Source: CAD feature listing. Evaluate the final solid. Frame: model axes, mm. Face numbers are marked on the shaded views. Give positions to 0.01 mm unless a question says otherwise; leave off trailing zeros. Loops run counter-clockwise (first coordinate to the right, second up) from the corner with the lowest first, then second, coordinate; pieces in that order, holes last.
from build123d import *

# Parameters (mm, degrees)
SKETCH1_R           = 1.5
SKETCH1_R_2         = 1.75
SKETCH1_R_3         = 1.45
BOSS_EXTRUDE1_DEPTH = 15


with BuildPart() as part:
    # Sketch1 → Boss-Extrude1 (new body)
    with BuildSketch(Plane(origin=(0, 0, 0), x_dir=(1, 0, 0), z_dir=(0, 1, 0))):
        with BuildLine():
            ThreePointArc((-2.52975, 1.612564708), (-7.95, 0), (-2.52975, -1.612564708))
            ThreePointArc((-2.52975, -1.612564708), (-0.159877177, -2.995736852), (2.34375, -1.872654783))
            ThreePointArc((2.34375, -1.872654783), (8.25, 0), (2.34375, 1.872654783))
            ThreePointArc((2.34375, 1.872654783), (-0.159877177, 2.995736852), (-2.52975, 1.612564708))
        make_face()
        with Locations(Location((0, 0, 0), (0, 0, 270))):
            Circle(SKETCH1_R, mode=Mode.SUBTRACT)
        with Locations(Location((5, 0, 0), (0, 0, 270))):
            Circle(SKETCH1_R_2, mode=Mode.SUBTRACT)
        with Locations(Location((-5, 0, 0), (0, 0, 270))):
            Circle(SKETCH1_R_3, mode=Mode.SUBTRACT)
    extrude(amount=BOSS_EXTRUDE1_DEPTH)


solid = part.part
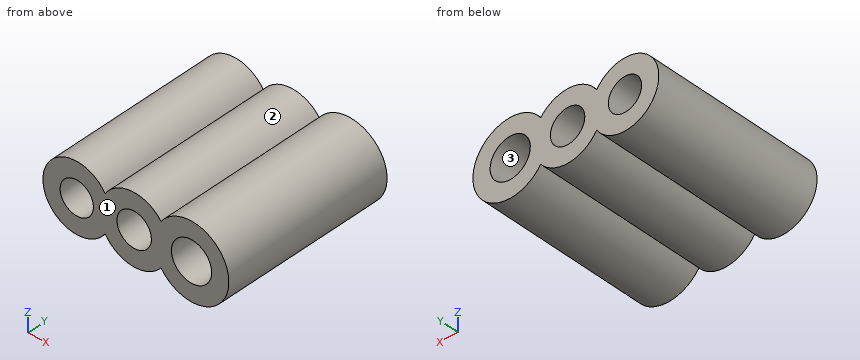
1) Cut plane C-C (y = 3). Return loops of the section in (x, z).
Checks:
outline: (-2.53, -1.61) arc R3 ccw to (2.34, -1.87) arc R3.25 ccw (long way) to (2.34, 1.87) arc R3 ccw to (-2.53, 1.61) arc R2.95 ccw (long way) to start; hole circle Ø2.9 at (-5, 0); hole circle Ø3 at (0, 0); hole circle Ø3.5 at (5, 0)
2) Ray query, probe 1 along X at (y, z) = (3.75, 0); probe 2 along X at (y, z) = (6.75, 1.25); probe 3 along X at (y, z) = (14, 2.25). Return the intervals inside material, ascending.
Checks:
probe 1: x = -7.95 to -6.45, -3.55 to -1.5, 1.5 to 3.25, 6.75 to 8.25
probe 2: x = -7.67 to -5.73, -4.27 to -0.83, 0.83 to 3.78, 6.22 to 8
probe 3: x = -6.91 to -3.09, -1.98 to 1.98, 2.65 to 7.35
3) Pull-direction query (X, two-part tool) for the marked faces 1, 2 and 3; classes: released by +X, released by -X, zero draft, split by the parting line, or undercut.
Checks:
face 1: zero draft
face 2: undercut
face 3: undercut
4) Cut plane B-B (z = 0). Return loops of the section in (x, y), and give its area (3 significant figures).
Checks:
outline: (-7.95, 0) - (-6.45, 0) - (-6.45, 15) - (-7.95, 15) - close; (-3.55, 0) - (-1.5, 0) - (-1.5, 15) - (-3.55, 15) - close; (1.5, 0) - (3.25, 0) - (3.25, 15) - (1.5, 15) - close; (6.75, 0) - (8.25, 0) - (8.25, 15) - (6.75, 15) - close
area: 102 mm2
5) Cut plane D-D (z = 2.25). Return loops of the section in (x, y).
Checks:
outline: (-6.91, 0) - (-3.09, 0) - (-3.09, 15) - (-6.91, 15) - close; (-1.98, 0) - (1.98, 0) - (1.98, 15) - (-1.98, 15) - close; (2.65, 0) - (7.35, 0) - (7.35, 15) - (2.65, 15) - close
6) Contact query for flat-ended pins moving along their axis: P1, Ø6, axis at x = -0.5, y = 7, coming from the +Z side; P2, Ø4, axis at x = -5.5, y = 8, coming from the +Z side; P3, Ø2.5, axis at x = -5, z = 0, coming from the +Y side. Output: stop coordinate, or through.
Checks:
P1: stops at z = 3
P2: stops at z = 2.95
P3: passes through
7) Cut plane A-A (x = -5). Return loops of the section in (y, z), and give its area (3 significant figures).
Checks:
outline: (0, -2.95) - (15, -2.95) - (15, -1.45) - (0, -1.45) - close; (0, 1.45) - (15, 1.45) - (15, 2.95) - (0, 2.95) - close
area: 45.0 mm2
